Check sheet for the drawn part. Datum: minimum x, y, z corner. Units: mm. A direction names the side the tool comes from. Round coordinates to 2 decimals unless told otherwise and drop trailing zeros. Write each loop counter-clockwise with the first axis right and the second up, starting at its lowest first coordinate (ties: lowest second). Pieces come first, ordered by that corner, then holes.
Item 1: Cross-section at C-C on x = 50. Enter the section's corners in (y, z).
Item 2: Cross-section at D-D on y = 19. Enter the section's corners in (x, z).
Item 3: Cross-section at B-B on z = 30. Enter the section's corners in (x, y).
Item 4: Material ranges on line 1 (X direction, y = 8, z = 30); line 2 (Y direction, x = 36.5, z = 12.5); line 3 (Z direction, x = 50, y = 11), recorded low to high.
Item 5: Tool access check on the marked faces 5, 6, 7, 8 and 9. Record the directions out of +Z, -Z, +X, -X, +Y, -Y that give a thin tool (end or side, any length) a straight path to the whole face; none if there is none.
Item 6: Cross-section at A-A on x = 113. Enter the section's corners in (y, z).
Item 7: Release check for a two-part mould opening along Z. For the marked faces 1, 2, 3 and 4 record: +Z half, -Z half, draft (parallel to the pull), parting line (faces both ways), or undercut.
Item 8: Go/stop test with flat-tipped pins: pin 1 Ø4.5 at (x, z) = (110, 50) entering from +Y; pin 2 Ø15 at (x, y) = (96, 29) entering from -Z; pin 3 Ø1.5 at (y, z) = (33.5, 49) entering from +X. Record where each tip stops, or that it passes through.
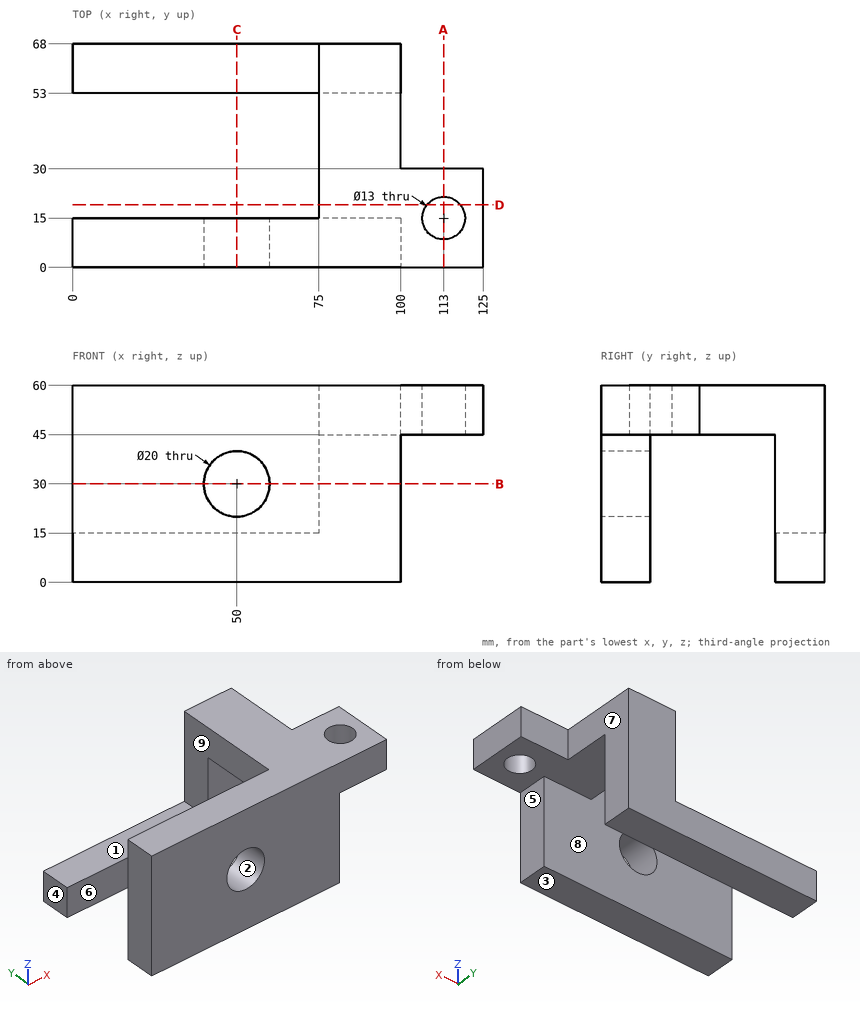
Response values:
1. outline: (0, 0) - (15, 0) - (15, 20) - (0, 20) - close; (0, 40) - (15, 40) - (15, 60) - (0, 60) - close; (53, 0) - (68, 0) - (68, 15) - (53, 15) - close
2. outline: (75, 45) - (107.88, 45) - (107.88, 60) - (75, 60) - close; (118.12, 45) - (125, 45) - (125, 60) - (118.12, 60) - close
3. outline: (0, 0) - (40, 0) - (40, 15) - (0, 15) - close; (60, 0) - (100, 0) - (100, 15) - (60, 15) - close; (75, 53) - (100, 53) - (100, 68) - (75, 68) - close
4. line 1: x = 0 to 40, 60 to 100
4. line 2: y = 0 to 15, 53 to 68
4. line 3: z = 0 to 20, 40 to 60
5. face 5: -Z, +X, +Y, -Y
5. face 6: -Z, +X, -X
5. face 7: +Z, -Z, +X, +Y
5. face 8: -Z, -X
5. face 9: +Z, -X, +Y
6. outline: (0, 45) - (8.5, 45) - (8.5, 60) - (0, 60) - close; (21.5, 45) - (30, 45) - (30, 60) - (21.5, 60) - close
7. face 1: +Z half
7. face 2: undercut
7. face 3: -Z half
7. face 4: draft
8. pin 1: stops at y = 30
8. pin 2: stops at z = 45
8. pin 3: stops at x = 100
